```python
from build123d import *

# Parameters (mm, degrees)
SKETCH1_R               = 5
SKETCH1_R_2             = 3.1
BOSS_EXTRUDE1_DEPTH     = 15
SKETCH2_R               = 5
BOSS_EXTRUDE2_DEPTH     = 1
BOSS_EXTRUDE3_DEPTH     = 10
SKETCH5_R               = 1.75
CUT_EXTRUDE1_DEPTH      = 28.26261176
CUT_EXTRUDE2_DEPTH      = 27.944387171
CUT_EXTRUDE2_DEPTH_BACK = 27.944387171


with BuildPart() as part:
    # Sketch1 → Boss-Extrude1 (new body)
    with BuildSketch(Plane(origin=(0, 0, 0), x_dir=(1, 0, 0), z_dir=(0, 1, 0))):
        with Locations(Location((0, 0, 0), (0, 0, 270))):
            Circle(SKETCH1_R)
        with Locations(Location((0, 0, 0), (0, 0, 270))):
            Circle(SKETCH1_R_2, mode=Mode.SUBTRACT)
    extrude(amount=BOSS_EXTRUDE1_DEPTH)

    # Sketch2 → Boss-Extrude2 (add)
    with BuildSketch(Plane(origin=(0, 15, 0), x_dir=(1, 0, 0), z_dir=(0, 1, 0))):
        with Locations(Location((0, 0, 0), (0, 0, 270))):
            Circle(SKETCH2_R)
    extrude(amount=BOSS_EXTRUDE2_DEPTH)

    # Sketch4 → Boss-Extrude3 (add)
    with BuildSketch(Plane(origin=(0, 16, 0), x_dir=(1, 0, 0), z_dir=(0, 1, 0))):
        with BuildLine():
            Line((-1.5, 4.769696007), (-1.5, -4.769696007))
            ThreePointArc((-1.5, -4.769696007), (0, -5), (1.5, -4.769696007))
            Line((1.5, -4.769696007), (1.5, 4.769696007))
            ThreePointArc((1.5, 4.769696007), (0, 5), (-1.5, 4.769696007))
        make_face()
    extrude(amount=BOSS_EXTRUDE3_DEPTH)

    # Sketch5 → Cut-Extrude1 (cut, through all)
    with BuildSketch(Plane.ZY.offset(1.5)):
        with Locations((0, 21)):
            Circle(SKETCH5_R)
    extrude(amount=-CUT_EXTRUDE1_DEPTH, mode=Mode.SUBTRACT)

    # Sketch6 → Cut-Extrude2 (cut, two sides: drawn at the far end of the back side and taken through both)
    with BuildSketch(Plane(origin=(0, 0, 0), x_dir=(0, 0, -1), z_dir=(1, 0, 0)).offset(-CUT_EXTRUDE2_DEPTH_BACK)):
        with BuildLine():
            Line((-5, 21), (-5, 26.951981281))
            Line((-5, 26.951981281), (5, 26.951981281))
            Line((5, 26.951981281), (5, 21))
            ThreePointArc((5, 21), (0, 26), (-5, 21))
        make_face()
    extrude(amount=CUT_EXTRUDE2_DEPTH + CUT_EXTRUDE2_DEPTH_BACK, mode=Mode.SUBTRACT)


solid = part.part
```
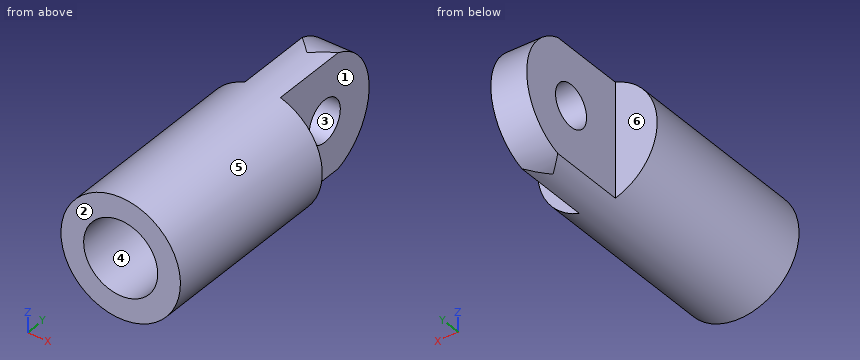
Build history of the part. All positions in model axes, mm. Face numbers are marked on the shaded views. A direction names the side the tool comes from. Coordinates: 2 decimals unless noted, no trailing zeros. Write each loop counter-clockwise with the first axis right and the second up, starting at its lowest first coordinate (ties: lowest second). Pieces come first, ordered by that corner, then holes.
1. 3-axis set-ups, long thin cutter, end or side, ignore diameter. For the marked faces 4, 5 and 6: which of +Z, -Z, +X, -X, +Y, -Y reach the whole face in a straight line?
Answer block:
face 4: -Y
face 5: +Y, -Y
face 6: +Z, -Z, -X, +Y
2. Band-saw the part on B-B, the plane x = 0. Give the cut face in (y, z).
Answer block:
outline: (0, -5) - (21, -5) arc R5 ccw to (21, 5) - (0, 5) - (0, 3.1) - (15, 3.1) - (15, -3.1) - (0, -3.1) - close; hole circle Ø3.5 at (21, 0)
3. Pull direction Y, two halves, no side cores. Call the marked faces 1, 2 and 3: released by +Y, released by -Y, zero draft, split by the parting line, or undercut.
Answer block:
face 1: zero draft
face 2: released by -Y
face 3: undercut
4. Band-saw the part on A-A, the plane z = 0. Give the cut face in (x, y), and give its area (3 significant figures).
Answer block:
outline: (-5, 0) - (-3.1, 0) - (-3.1, 15) - (3.1, 15) - (3.1, 0) - (5, 0) - (5, 16) - (1.5, 16) - (1.5, 19.25) - (-1.5, 19.25) - (-1.5, 16) - (-5, 16) - close; (-1.5, 22.75) - (1.5, 22.75) - (1.5, 26) - (-1.5, 26) - close
area: 86.5 mm2
5. Band-saw the part on C-C, the plane y = 7. Give the cut face in (x, z).
Answer block:
outline: circle Ø10 at (0, 0); hole circle Ø6.2 at (0, 0)
6. Band-saw the part on D-D, the plane z = 2.5. Give the cut face in (x, y).
Answer block:
outline: (-4.33, 0) - (-1.83, 0) - (-1.83, 15) - (1.83, 15) - (1.83, 0) - (4.33, 0) - (4.33, 16) - (1.5, 16) - (1.5, 25.33) - (-1.5, 25.33) - (-1.5, 16) - (-4.33, 16) - close
7. Drop flat-ended pins along their axis: pin 1 (2 mm diameter, centred on y = 6, z = 0.5, fed in from -X); pin 2 (3 mm diameter, centred on x = -1, z = 1, fed in from -Y); pin 3 (3 mm diameter, centred on x = 3.5, z = -0.5, fed in from +Y); pin 4 (3 mm diameter, centred on x = 2.5, z = 1.5, fed in from +Y). Give the stop position or say it passes through.
Answer block:
pin 1: stops at x = -5
pin 2: stops at y = 15
pin 3: stops at y = 16
pin 4: stops at y = 25.99
8. Drill centre lines: probe 1 along X at (y, z) = (6, 0); probe 2 along Y at (x, z) = (0.8, 0); probe 3 along X at (y, z) = (17, -4). Where is each one in solid material? Low to high.
Answer block:
probe 1: x = -5 to -3.1, 3.1 to 5
probe 2: y = 15 to 19.25, 22.75 to 26
probe 3: x = -1.5 to 1.5
